from build123d import *

# Parameters (mm, degrees)
F1_DEPTH      = 8
F2_R          = 2.5
F3_DEPTH      = 8.296516
F3_DEPTH_BACK = 8.296516


with BuildPart() as f1:
    # F0 (on Front) → F1 (new body)
    with BuildSketch(Plane.XZ):
        with BuildLine():
            Line((20.080229, 8.296516), (-20.080229, 8.296516))
            ThreePointArc((-20.080229, 8.296516), (-25.793151, 5.783339), (-28.139749, 0))
            Line((-28.139749, 0), (-22.095229, 0))
            ThreePointArc((-22.095229, 0), (-20.080229, 2.015), (-18.065229, 0))
            Line((-18.065229, 0), (18.065229, 0))
            ThreePointArc((18.065229, 0), (20.080229, 2.015), (22.095229, 0))
            Line((22.095229, 0), (28.376744, 0))
            ThreePointArc((28.376744, 0), (25.946751, 5.866522), (20.080229, 8.296516))
        make_face()
        with BuildLine():
            Line((-22.095229, 0), (-28.139749, 0))
            ThreePointArc((-28.139749, 0), (-25.793151, -5.783339), (-20.080229, -8.296516))
            Line((-20.080229, -8.296516), (20.080229, -8.296516))
            ThreePointArc((20.080229, -8.296516), (25.946751, -5.866522), (28.376744, 0))
            Line((28.376744, 0), (22.095229, 0))
            ThreePointArc((22.095229, 0), (20.080229, -2.015), (18.065229, 0))
            Line((18.065229, 0), (-18.065229, 0))
            ThreePointArc((-18.065229, 0), (-20.080229, -2.015), (-22.095229, 0))
        make_face()
    extrude(amount=F1_DEPTH)

    # F2 (on Top) → F3 (join, two sides)
    with BuildSketch(Plane.XY) as f3_sk:
        with BuildLine():
            Line((-13.025831, 0), (13.025831, 0))
            ThreePointArc((13.025831, 0), (0, 12.5), (-13.025831, 0))
        make_face()
        with Locations((0, 7.5)):
            Circle(F2_R, mode=Mode.SUBTRACT)
    extrude(amount=F3_DEPTH)
    extrude(f3_sk.sketch, amount=-F3_DEPTH_BACK)


solid = f1.part
For this review, take the finished solid that the model builds, in its own axes (mm). A direction names the side the tool comes from. Coordinates: 2 decimals unless noted, no trailing zeros. Order: outer loops, then holes, each group sorted by start corner. A loop starts at its lowest first (then second) coordinate and runs counter-clockwise, first axis right, second up. Notation, with made-up numbers: (79, 14) -> (102, 14) arc R32 ccw to (102, 47) -> close; hole circle Ø10 at (82.25, -33). An arc over 180 degrees is marked (long way). Return JSON: item names as keys, results as strings.
1. The part is to be moulded in two halves that separate along Z. For faces 1 (the cylindrical face through (-22.093, -3.944, -0.089)), 2 (the flat face through (0, 0, 8.297)), 3 (the cylindrical face through (-0.54, 5.06, -0.12)), say which applies: +Z half, -Z half, draft (parallel to the pull), parting line (faces both ways), or undercut.
Answer block:
{"face 1": "undercut", "face 2": "+Z half", "face 3": "draft"}
2. For pin 1 Ø5 at (x, z) = (-6, 1.5) entering from +Y; pin 2 Ø12 at (x, y) = (-20, 10) entering from +Z; pin 3 Ø4 at (x, z) = (20.5, -3.5) entering from +Y, all flat-tipped, find the tip position at first contact; note any pin that passes through.
Answer block:
{"pin 1": "y = 12.02", "pin 2": "through", "pin 3": "y = 0"}
3. We need section C-C on y = 7.5. Write out the cut boundary in (x, z).
Answer block:
{"outline": "(-10.26, -8.3) -> (-2.5, -8.3) -> (-2.5, 8.3) -> (-10.26, 8.3) -> close; (2.5, -8.3) -> (10.26, -8.3) -> (10.26, 8.3) -> (2.5, 8.3) -> close"}
4. Machinability: for faces 4 (the flat face through (21, 0, 2)), 5 (the cylindrical face through (22, -3.94, -0.61)), 6 (the flat face through (-21, 0, 2)), which of the approach directions +Z, -Z, +X, -X, +Y, -Y give a long, thin tool a straight path to every point of the face, cutting with its end or side? Answer none if there is none.
Answer block:
{"face 4": "+Z, -Z, +X, +Y", "face 5": "+Y, -Y", "face 6": "+Z, -Z, -X, +Y"}
5. For line 1 (Y direction, x = 25, z = 1.25); line 2 (Z direction, x = 21.5, y = -1); line 3 (Y direction, x = -9, z = -1.25) (3 decimals), list the stretches that pass through material, from the lowest coordinate up. Write a range as from..to.
Answer block:
{"line 1": "-8..0", "line 2": "-8.17..-1.43, 1.43..8.17", "line 3": "-8..8.895"}
6. We need section D-D on z = 3.5. Write out the cut boundary in (x, y), and give its area (3 significant figures).
Answer block:
{"outline": "(-27.37, -8) -> (27.6, -8) -> (27.6, 0) -> (13.03, 0) arc R13.04 ccw to (-13.03, 0) -> (-27.37, 0) -> close; hole circle Ø5 at (0, 7.5)", "area": "673 mm²"}
7. We need section B-B on y = -1. Write out the cut boundary in (x, z) (3 decimals).
Answer block:
{"outline": "(-20.08, -8.297) -> (20.08, -8.297) arc R8.297 ccw to (28.377, 0) arc R8.297 ccw to (20.08, 8.297) -> (-20.08, 8.297) arc R8.3 ccw to start; hole circle Ø4.03 at (-20.08, 0); hole circle Ø4.03 at (20.08, 0)"}
8. We need section A-A on x = 0. Write out the cut boundary in (y, z).
Answer block:
{"outline": "(-8, -8.3) -> (5, -8.3) -> (5, 8.3) -> (-8, 8.3) -> close; (10, -8.3) -> (12.5, -8.3) -> (12.5, 8.3) -> (10, 8.3) -> close"}
